Here's the drawing with two shaded views (mm, measured from the low corner). I have some questions. A direction names the side the tool comes from. Coordinates: 2 decimals unless noted, no trailing zeros. Loops run counter-clockwise (first coordinate to the right, second up) from the corner with the lowest first, then second, coordinate; pieces in that order, holes last.
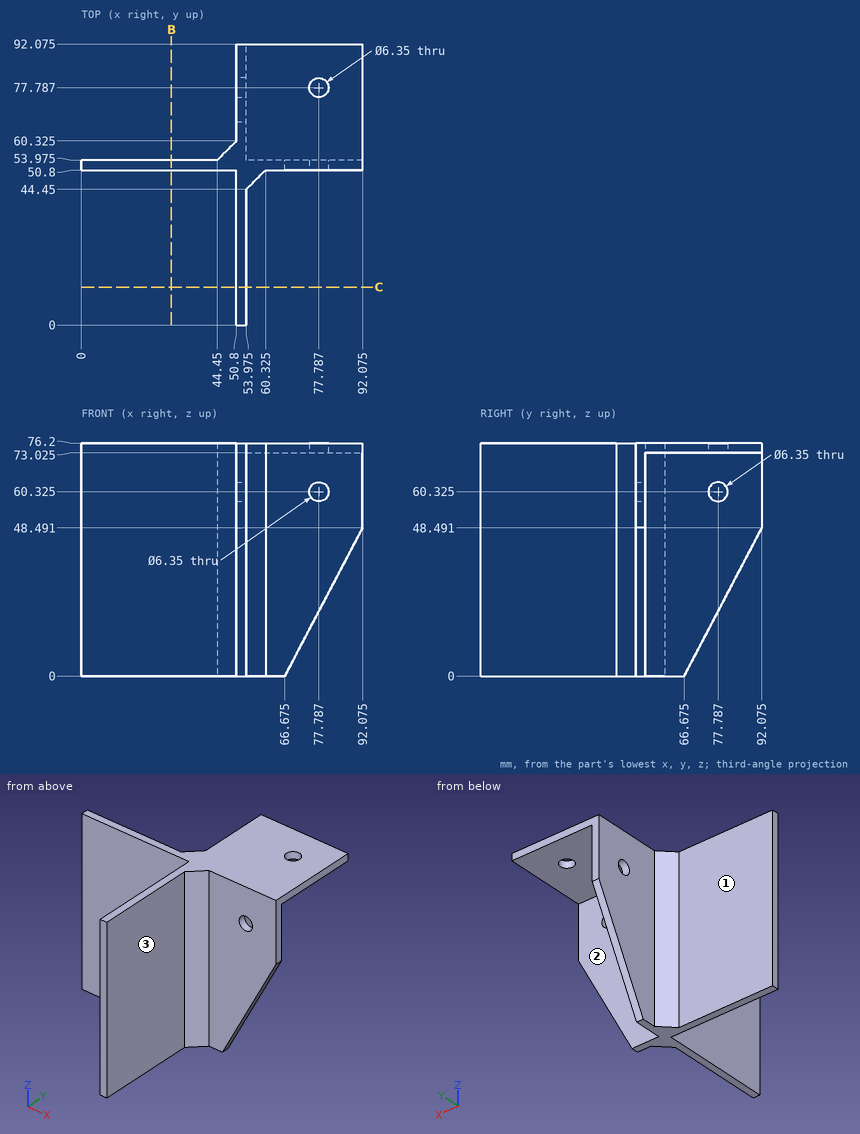
Q1. Suppose I cut it at B-B on x = 29.5. Write out the boundary of the cut face in (y, z) (1 decimal).
Q2. Will these pins go through, and if not, where does the flat tip stop? P1, Ø3, axis at x = 12.5, z = 36, coming from the +Y side (1 decimal); P2, Ø2, axis at y = 21, z = 42.5, coming from the +X side (1 decimal); P3, Ø8, axis at x = 47, z = 48, coming from the -Y side; P4, Ø10, axis at x = 77.79, y = 77.79, coming from the -Z side (1 decimal).
Q3. Please list where these lines run through material, in increasing order: probe 1 along X at (y, z) = (39, 43) (1 decimal); probe 2 along Z at (x, y) = (68.5, 63.5) (1 decimal).
Q4. For the marked faces 1, 2 and 3, which set-ups out of +Z, -Z, +X, -X, +Y, -Y let a thin tool reach every point of the face, with its end or its side?
Check values:
1. outline: (50.8, 0) - (54, 0) - (54, 76.2) - (50.8, 76.2) - close
2. P1: stops at y = 54
2. P2: stops at x = 54
2. P3: stops at y = 0
2. P4: stops at z = 73
3. probe 1: x = 50.8 to 54
3. probe 2: z = 73 to 76.2
4. face 1: +Z, -Z, -X, +Y
4. face 2: -Z, +X, +Y
4. face 3: +Z, -Z, +X, -Y
